```python
from build123d import *

# Parameters (mm, degrees)
BOSS_EXTRUDE1_DEPTH     = 15
SKETCH3_R               = 7.5
SKETCH2_R               = 10
SKETCH4_R               = 2.5
CUT_EXTRUDE1_DEPTH      = 22.0000001
CUT_EXTRUDE1_DEPTH_BACK = 1


with BuildPart() as part:
    # Sketch1 → Boss-Extrude1 (new body)
    with BuildSketch(Plane(origin=(0, 0, 0), x_dir=(1, 0, 0), z_dir=(0, 1, 0))):
        with BuildLine():
            Line((-6.32455532, -3), (-4, -3))
            Line((-4, -3), (-4, 3))
            Line((-4, 3), (-6.32455532, 3))
            ThreePointArc((-6.32455532, 3), (0, 7), (6.32455532, 3))
            Line((6.32455532, 3), (4, 3))
            Line((4, 3), (4, -3))
            Line((4, -3), (6.32455532, -3))
            ThreePointArc((6.32455532, -3), (0, -7), (-6.32455532, -3))
        make_face()
    extrude(amount=BOSS_EXTRUDE1_DEPTH)

    # Sketch3 → Loft1 section 0
    with BuildSketch(Plane(origin=(0, 23, 0), x_dir=(1, 0, 0), z_dir=(0, 1, 0))):
        Circle(SKETCH3_R)
    # Sketch2 → Loft1 section 1
    with BuildSketch(Plane(origin=(0, 15, 0), x_dir=(1, 0, 0), z_dir=(0, 1, 0))):
        Circle(SKETCH2_R)
    loft()

    # Sketch4 → Cut-Extrude1 (cut, two sides)
    with BuildSketch(Plane.XY.offset(-11)) as cut_extrude1_sk:
        with Locations((0, 6)):
            Circle(SKETCH4_R)
    extrude(amount=CUT_EXTRUDE1_DEPTH, mode=Mode.SUBTRACT)
    extrude(cut_extrude1_sk.sketch, amount=-CUT_EXTRUDE1_DEPTH_BACK, mode=Mode.SUBTRACT)


solid = part.part
```
Verification items for the finished model (mm, model axes). A direction names the side the tool comes from. Give positions to 0.01 mm unless a question says otherwise; leave off trailing zeros. Order: outer loops, then holes, each group sorted by start corner. A loop starts at its lowest first (then second) coordinate and runs counter-clockwise, first axis right, second up. Notation, with made-up numbers: M 37.5,23.25 L 41.5,23.25 A12 ccw 41.5,27.25 Z; hole C 23,8.5 d7. An arc over 180 degrees is marked long. Answer in a Markdown table with one row per item. Add a question column.
Item 1: Tool access check on faces 1 (the cylindrical face through (0, 9, -7)), 2 (the flat face through (0, 0, 0)), 3 (the flat face through (5, 7, 3)), 4 (the flat face through (-4, 7, 0)), 5 (the cylindrical face through (0, 9, 7)). Record the directions out of +Z, -Z, +X, -X, +Y, -Y that give a thin tool (end or side, any length) a straight path to the whole face; none if there is none.
Item 2: Mould release check, pull along Z, two halves, no side actions. Record for faces 6 (the flat face through (-5, 7, 3)), 7 (the conical face through (-5.85, 21.61, -5.36)), 8 (the cylindrical face through (-0.33, 8.48, -0.1)): released by +Z, released by -Z, zero draft, split by the parting line, or undercut.
Item 3: Section check A-A, the plane x = 0. Enter the section's corners in (y, z), and give its area (3 significant figures).
Item 4: Section check B-B, the plane y = 4.25. Enter the section's corners in (x, z).
Item 5: Section check C-C, the plane y = 12.5. Enter the section's corners in (x, z).
Item 6: Scan lines: probe 1 along Y at (x, z) = (0, -2.25); probe 2 along X at (y, z) = (6, 2.5); probe 3 along Z at (x, y) = (5, 12). Record each from-to range of solid material in increasing order. Write a range as from..to.
Item 7: Gauge pin test, flat ends, axial feed: pin 1 (0.7 mm diameter, centred on x = 5, y = 5, fed in from +Z); pin 2 (6.5 mm diameter, centred on y = 9.5, z = 1.5, fed in from +X); pin 3 (2.5 mm diameter, centred on x = -4.5, y = 11, fed in from +Z). Record the tip position at first contact, or that the pin passes through.
Filled sheet:
| question | item | result |
|---|---|---|
| 1 | face 1 | -Z, -Y |
| 1 | face 2 | +Z, -Z, +X, -X, -Y |
| 1 | face 3 | +X, -Y |
| 1 | face 4 | -X, -Y |
| 1 | face 5 | +Z, -Y |
| 2 | face 6 | undercut |
| 2 | face 7 | split by the parting line |
| 2 | face 8 | zero draft |
| 3 | outline | M 0,-7 L 3.5,-7 L 3.5,7 L 0,7 Z; M 8.5,-7 L 15,-7 L 15,-10 L 23,-7.5 L 23,7.5 L 15,10 L 15,7 L 8.5,7 Z |
| 3 | area | 280 mm^2 |
| 4 | outline | M -6.32,-3 A7 ccw -1.79,-6.77 L -1.79,6.77 A7 ccw -6.32,3 L -4,3 L -4,-3 Z; M 1.79,-6.77 A7 ccw 6.32,-3 L 4,-3 L 4,3 L 6.32,3 A7 ccw 1.79,6.77 Z |
| 5 | outline | M -6.32,-3 A7 ccw 6.32,-3 L 4,-3 L 4,3 L 6.32,3 A7 ccw -6.32,3 L -4,3 L -4,-3 Z |
| 6 | probe 1 | y = 0..3.5, 8.5..23 |
| 6 | probe 2 | x = -4..-2.5, 2.5..4 |
| 6 | probe 3 | z = -4.9..-3, 3..4.9 |
| 7 | pin 1 | stops at z = 5.23 |
| 7 | pin 2 | stops at x = 6.32 |
| 7 | pin 3 | stops at z = 6.2 |
